The drawing under review shows one solid part. Ordinate dimensions are in mm from its lowest x, y, z. A direction names the side the tool comes from. Coordinates: 2 decimals unless noted, no trailing zeros. Order: outer loops, then holes, each group sorted by start corner. A loop starts at its lowest first (then second) coordinate and runs counter-clockwise, first axis right, second up.
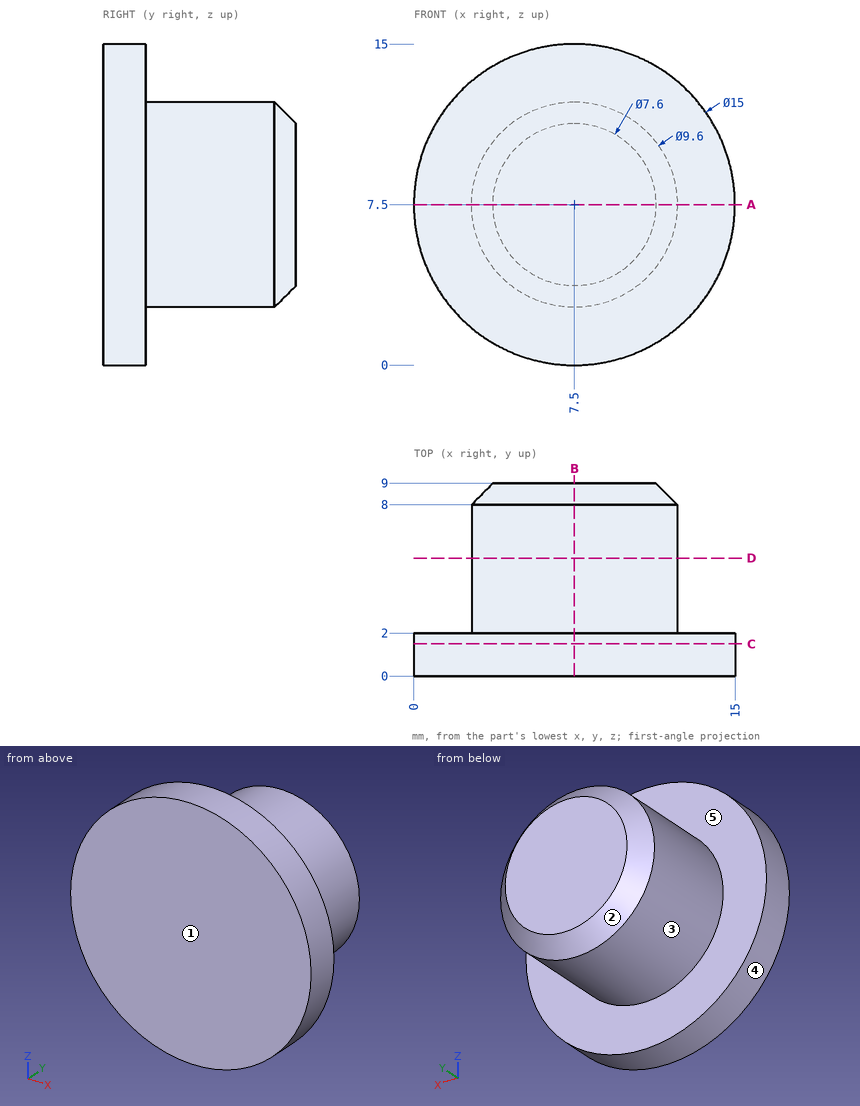
(1) We need section A-A, the plane z = 7.5. Write out the cut boundary in (x, y).
A:
outline: (0, 0) - (15, 0) - (15, 2) - (12.3, 2) - (12.3, 8) - (11.3, 9) - (3.7, 9) - (2.7, 8) - (2.7, 2) - (0, 2) - close
(2) Draft analysis for pull direction Y (two halves, no side actions). For the marked faces 1, 2 and 3, state which applies: released by +Y, released by -Y, zero draft, split by the parting line, or undercut.
A:
face 1: released by -Y
face 2: released by +Y
face 3: zero draft
(3) Machinability: for the marked faces 4 and 5, which of the approach directions +Z, -Z, +X, -X, +Y, -Y give a long, thin tool a straight path to every point of the face, cutting with its end or side? Answer none if there is none.
A:
face 4: +Y, -Y
face 5: +Y
(4) For pin 1 Ø5 at (x, z) = (12.5, 12.5) entering from +Y; pin 2 Ø1 at (x, y) = (13, 4.5) entering from -Z; pin 3 Ø2 at (x, z) = (6.5, 2.5) entering from +Y, all flat-tipped, find the tip position at first contact; note any pin that passes through.
A:
pin 1: stops at y = 8.23
pin 2: passes through
pin 3: stops at y = 8.7
(5) Wall thickness on probe 1 along Y at (x, z) = (8.75, 14); probe 2 along Z at (x, y) = (6.75, 1.5); probe 3 along Z at (x, y) = (6, 1.5): over which ranges is each line inside the solid? List them lowest first.
A:
probe 1: y = 0 to 2
probe 2: z = 0.04 to 14.96
probe 3: z = 0.15 to 14.85
(6) We need section C-C, the plane y = 1.5. Write out the cut boundary in (x, z).
A:
outline: circle Ø15 at (7.5, 7.5)
(7) We need section D-D, the plane y = 5.5. Write out the cut boundary in (x, z).
A:
outline: circle Ø9.6 at (7.5, 7.5)
(8) We need section B-B, the plane x = 7.5. Write out the cut boundary in (y, z).
A:
outline: (0, 0) - (2, 0) - (2, 2.7) - (8, 2.7) - (9, 3.7) - (9, 11.3) - (8, 12.3) - (2, 12.3) - (2, 15) - (0, 15) - close
